from build123d import *

# Parameters (mm, degrees)
BOSS_EXTRUDE1_DEPTH = 3.048
SKETCH2_W           = 10.16
SKETCH2_H           = 3.175
CUT_EXTRUDE1_DEPTH  = 54.967678327


with BuildPart() as part:
    # Sketch1 → Boss-Extrude1 (new body)
    with BuildSketch(Plane(origin=(0, 0, 0), x_dir=(1, 0, 0), z_dir=(0, 1, 0))):
        with BuildLine():
            Line((3.175, 38.1), (3.175, 26.67))
            Line((3.175, 26.67), (0, 26.67))
            Line((0, 26.67), (0, 19.850704534))
            ThreePointArc((0, 19.850704534), (3.3655, 19.05), (0, 18.249295466))
            Line((0, 18.249295466), (0, 11.43))
            Line((0, 11.43), (3.175, 11.43))
            Line((3.175, 11.43), (3.175, 0))
            Line((3.175, 0), (34.925, 0))
            Line((34.925, 0), (34.925, 11.43))
            Line((34.925, 11.43), (38.1, 11.43))
            Line((38.1, 11.43), (38.1, 18.249295466))
            ThreePointArc((38.1, 18.249295466), (34.7345, 19.05), (38.1, 19.850704534))
            Line((38.1, 19.850704534), (38.1, 26.67))
            Line((38.1, 26.67), (34.925, 26.67))
            Line((34.925, 26.67), (34.925, 38.1))
            Line((34.925, 38.1), (3.175, 38.1))
        make_face()
    extrude(amount=BOSS_EXTRUDE1_DEPTH)

    # Sketch2 → Cut-Extrude1 (cut, through all)
    with BuildSketch(Plane(origin=(0, 3.048, 0), x_dir=(1, 0, 0), z_dir=(0, 1, 0))):
        with Locations((19.05, 2.8575)):
            Rectangle(SKETCH2_W, SKETCH2_H)
    extrude(amount=-CUT_EXTRUDE1_DEPTH, mode=Mode.SUBTRACT)


solid = part.part
The listing builds one solid part. Answer for the finished solid, in the listing's coordinates (mm). A direction names the side the tool comes from. Give positions to 0.01 mm unless a question says otherwise; leave off trailing zeros. Write each loop counter-clockwise with the first axis right and the second up, starting at its lowest first coordinate (ties: lowest second). Pieces come first, ordered by that corner, then holes.
1) Given P1, Ø0.9, axis at y = 2, z = -7, coming from the -X side (3 decimals); P2, Ø1.5, axis at y = 1.5, z = -32.5, coming from the +X side (3 decimals); P3, Ø1.5, axis at x = 36.5, y = 1, coming from the +Z side, each flat-ended and moving along its own axis, determine where each tip first touches the part or whether it passes through.
2) Section A-A (z = -3) is taken. Write down the section's boundary in (x, y) (3 decimals).
3) Find the intervals of material crossed by L1, parallel to Z at x = 20, y = 1.25 (3 decimals); L2, parallel to X at y = 2.3, z = -19.05; L3, parallel to X at y = 0.25, z = -18, in increasing order.
4) Section C-C (x = 22) is taken. Write down the section's boundary in (y, z) (3 decimals).
5) A tool of negligible diameter and unlimited length cuts with its end or side. For faces 1 (the face through (36, 2, -11.43)), 2 (the face through (24.13, 2, -3)), 3 (the face through (3.175, 2, -6)), 4 (the face through (34.925, 2, -32)), 5 (the face through (3.175, 2, -32)), from which of +Z, -Z, +X, -X, +Y, -Y can it reach the whole face along a straight path? Write none if from no direction.
6) Section D-D (z = -19.05) is taken. Write down the section's boundary in (x, y), and give its area (3 significant figures).
7) For a pull along Z with two mould halves and no side action, classify faces 6 (the face through (19, 3.048, -19)), 7 (the face through (37, 2, -26.67)), 8 (the face through (19, 2, -4.445)), 9 (the face through (19, 2, -1.27)) as pulls with the +Z half, pulls with the -Z half, needs draft (parallel to the pull), parting line crosses it, or undercut.
Response:
1. P1: stops at x = 3.175
1. P2: stops at x = 34.925
1. P3: stops at z = -11.43
2. outline: (3.175, 0) - (13.97, 0) - (13.97, 3.048) - (3.175, 3.048) - close; (24.13, 0) - (34.925, 0) - (34.925, 3.048) - (24.13, 3.048) - close
3. L1: z = -38.1 to -4.445, -1.27 to 0
3. L2: x = 3.37 to 34.73
3. L3: x = 0 to 0.15, 3.02 to 35.08, 37.95 to 38.1
4. outline: (0, -38.1) - (3.048, -38.1) - (3.048, -4.445) - (0, -4.445) - close; (0, -1.27) - (3.048, -1.27) - (3.048, 0) - (0, 0) - close
5. face 1: +Z, +X, +Y, -Y
5. face 2: +Y, -Y
5. face 3: +Z, -X, +Y, -Y
5. face 4: -Z, +X, +Y, -Y
5. face 5: -Z, -X, +Y, -Y
6. outline: (3.37, 0) - (34.73, 0) - (34.73, 3.05) - (3.37, 3.05) - close
6. area: 95.6 mm2
7. face 6: needs draft
7. face 7: pulls with the -Z half
7. face 8: undercut
7. face 9: undercut
